Check sheet for the modelled part. Datum: model origin and axes. Units: mm. A direction names the side the tool comes from. Round coordinates to 2 decimals unless told otherwise and drop trailing zeros. Write each loop counter-clockwise with the first axis right and the second up, starting at its lowest first coordinate (ties: lowest second). Pieces come first, ordered by that corner, then holes. Notation, with made-up numbers: (-2, 38.25) -> (32, 38.25) arc R19 cw to (32, 75.25) -> close; hole circle Ø9 at (0, 21). An arc over 180 degrees is marked (long way). Write item = value, one per line.
from build123d import *

# Parameters (mm, degrees)
CROQUIS1_W              = 164.9
CROQUIS1_H              = 102
SALIENTE_EXTRUIR2_DEPTH = 14.27
CROQUIS2_W              = 174.9
CROQUIS2_H              = 112
CROQUIS2_W_2            = 166.9
CROQUIS2_H_2            = 104
SALIENTE_EXTRUIR3_DEPTH = 14.27
CROQUIS3_W              = 174.9
CROQUIS3_H              = 112
CROQUIS3_W_2            = 160.9
CROQUIS3_H_2            = 98.374406292
SALIENTE_EXTRUIR5_DEPTH = 1
CROQUIS4_W              = 164.9
CROQUIS4_H              = 102
CORTAR_EXTRUIR2_DEPTH   = 14.27
CROQUIS6_W              = 174.9
CROQUIS6_H              = 112
CROQUIS6_R              = 1.5
SALIENTE_EXTRUIR6_DEPTH = 15
CROQUIS8_W              = 160.9
CROQUIS8_H              = 98.374406292
CORTAR_EXTRUIR3_DEPTH   = 9
CROQUIS9_W              = 166.9
CROQUIS9_H              = 104
CORTAR_EXTRUIR5_DEPTH   = 11


with BuildPart() as part:
    # Croquis1 → Saliente-Extruir2 (new body)
    with BuildSketch(Plane(origin=(0, 0, 0), x_dir=(0, 0, -1), z_dir=(1, 0, 0))):
        Rectangle(CROQUIS1_W, CROQUIS1_H)
    extrude(amount=SALIENTE_EXTRUIR2_DEPTH)

    # Croquis4 → Cortar-Extruir2 (cut)
    with BuildSketch(Plane(origin=(14.27, 0, 0), x_dir=(0, 0, -1), z_dir=(1, 0, 0))):
        Rectangle(CROQUIS4_W, CROQUIS4_H)
    extrude(amount=-CORTAR_EXTRUIR2_DEPTH, mode=Mode.SUBTRACT)


with BuildPart() as body_2:
    # Croquis2 → Saliente-Extruir3 (new body)
    with BuildSketch(Plane(origin=(0, 0, 0), x_dir=(0, 0, -1), z_dir=(1, 0, 0))):
        Rectangle(CROQUIS2_W, CROQUIS2_H)
        Rectangle(CROQUIS2_W_2, CROQUIS2_H_2, mode=Mode.SUBTRACT)
    extrude(amount=SALIENTE_EXTRUIR3_DEPTH)

    # Croquis3 → Saliente-Extruir5 (add)
    with BuildSketch(Plane.ZY):
        Rectangle(CROQUIS3_W, CROQUIS3_H)
        with Locations((0, -0.062203146)):
            Rectangle(CROQUIS3_W_2, CROQUIS3_H_2, mode=Mode.SUBTRACT)
    extrude(amount=SALIENTE_EXTRUIR5_DEPTH)

    # Croquis6 → Saliente-Extruir6 (add)
    with BuildSketch(Plane(origin=(14.27, 0, 0), x_dir=(0, 0, -1), z_dir=(1, 0, 0))):
        Rectangle(CROQUIS6_W, CROQUIS6_H)
        with Locations((-77.445, 46)):
            Circle(CROQUIS6_R, mode=Mode.SUBTRACT)
        with Locations((-77.445, -46)):
            Circle(CROQUIS6_R, mode=Mode.SUBTRACT)
        with Locations((-22.1, 15.81)):
            Circle(CROQUIS6_R, mode=Mode.SUBTRACT)
        with Locations((35.9, 15.81)):
            Circle(CROQUIS6_R, mode=Mode.SUBTRACT)
        with Locations((-22.1, -33.19)):
            Circle(CROQUIS6_R, mode=Mode.SUBTRACT)
        with Locations((35.9, -33.19)):
            Circle(CROQUIS6_R, mode=Mode.SUBTRACT)
        with Locations((77.445, 46)):
            Circle(CROQUIS6_R, mode=Mode.SUBTRACT)
        with Locations((77.445, -46)):
            Circle(CROQUIS6_R, mode=Mode.SUBTRACT)
    extrude(amount=SALIENTE_EXTRUIR6_DEPTH)

    # Croquis8 → Cortar-Extruir3 (cut)
    with BuildSketch(Plane.ZY.offset(-14.27)):
        with Locations((0, -0.062203146)):
            Rectangle(CROQUIS8_W, CROQUIS8_H)
    extrude(amount=-CORTAR_EXTRUIR3_DEPTH, mode=Mode.SUBTRACT)

    # Croquis9 → Cortar-Extruir5 (cut)
    with BuildSketch(Plane.ZY.offset(-14.27)):
        Rectangle(CROQUIS9_W, CROQUIS9_H)
    extrude(amount=-CORTAR_EXTRUIR5_DEPTH, mode=Mode.SUBTRACT)


solid = body_2.part
(1) Sectioned sample at B-B on y = 2. Enter the section's corners in (x, z), then the cut area to 3 significant figures.
Worked answers:
outline = (-1, -87.45) -> (29.27, -87.45) -> (29.27, 87.45) -> (-1, 87.45) -> (-1, 80.45) -> (0, 80.45) -> (0, 83.45) -> (25.27, 83.45) -> (25.27, -83.45) -> (0, -83.45) -> (0, -80.45) -> (-1, -80.45) -> close
area = 916 mm²
(2) Go/stop test with flat-tipped pins: P1, Ø3.5, axis at y = 15.81, z = 22.1, coming from the -X side; P2, Ø2.5, axis at y = -33.19, z = 22.1, coming from the -X side. Record where each tip stops, or that it passes through.
Worked answers:
P1 = 25.27
P2 = through
(3) Release check for a two-part mould opening along Z. For faces 1 (the flat face through (14, -1, 87.45)), 2 (the flat face through (14, -56, 1)), 3 (the flat face through (12, -1, 83.45)) record: pulls with the +Z half, pulls with the -Z half, needs draft (parallel to the pull), parting line crosses it, or undercut.
Worked answers:
face_1 = pulls with the +Z half
face_2 = needs draft
face_3 = undercut
(4) Sectioned sample at A-A on x = 20. Enter the section's corners in (y, z), then the cut area to 3 significant figures.
Worked answers:
outline = (-56, -87.45) -> (56, -87.45) -> (56, 87.45) -> (-56, 87.45) -> close; hole (-52, -83.45) -> (52, -83.45) -> (52, 83.45) -> (-52, 83.45) -> close
area = 2,230 mm²
(5) Sectioned sample at C-C on z = 49. Enter the section's corners in (x, y) (3 decimals).
Worked answers:
outline = (-1, -56) -> (29.27, -56) -> (29.27, 56) -> (-1, 56) -> (-1, 49.125) -> (0, 49.125) -> (0, 52) -> (25.27, 52) -> (25.27, -52) -> (0, -52) -> (0, -49.249) -> (-1, -49.249) -> close
(6) Access from +Z, -Z, +X, -X, +Y, -Y to the whole of each face (thin tool, end or side, straight path). Record for faces 4 (the flat face through (12, -52, -1)), 5 (the flat face through (14, -1, -87.45)).
Worked answers:
face_4 = none
face_5 = -Z, +X, -X, +Y, -Y
(7) Material ranges on L1, parallel to Z at x = 27.1, y = -46 (3 decimals); L2, parallel to Y at x = 26.8, z = -35.9; L3, parallel to Z at x = 28.5, y = 15.81, recorded low to high. Write a range as [from, to].
Worked answers:
L1 = [-87.45, -78.945], [-75.945, 75.945], [78.945, 87.45]
L2 = [-56, -34.69], [-31.69, 14.31], [17.31, 56]
L3 = [-87.45, -37.4], [-34.4, 20.6], [23.6, 87.45]
